For this review, take the finished solid that the model builds, in its own axes (mm). A direction names the side the tool comes from. Round coordinates to 2 decimals unless told otherwise and drop trailing zeros. Order: outer loops, then holes, each group sorted by start corner. A loop starts at its lowest first (then second) coordinate and runs counter-clockwise, first axis right, second up.
Autodesk Inventor part; units mm, degrees
ref_plane "Work Plane1" through (0, 98, 0) normal (0, -1, 0) x (1, 0, 0)
ref_plane "YZ Plane" through (0, 0, 0) normal (1, 0, 0) x (0, 1, 0)
ref_plane "XZ Plane" through (0, 0, 0) normal (0, 1, 0) x (-1, 0, 0)
sketch "Sketch1" plane through (0, 0, 0) normal (0, 1, 0) x (-1, 0, 0)
  line L0 (0, 0) -> (8, 0)
  line L1 (8, 0) -> (8, -120)
  line L2 (8, -120) -> (0, -120)
  line L3 (0, -120) -> (0, 0)
  line L4 (8, 0) -> (38, 0)
  line L5 (38, 0) -> (38, -120)
  line L6 (38, -120) -> (8, -120)
  line L7 (8, -120) -> (8, 0)
  circle A0 centre (20, -17) radius 2
  circle A1 centre (20, -30) radius 2
  circle A2 centre (20, -43) radius 2
  circle A3 centre (20, -77) radius 2
  circle A4 centre (20, -90) radius 2
  circle A5 centre (20, -103) radius 2
  circle A6 centre (30, -17) radius 2
  circle A7 centre (30, -30) radius 2
  circle A8 centre (30, -43) radius 2
  circle A9 centre (30, -77) radius 2
  circle A10 centre (30, -90) radius 2
  circle A11 centre (30, -103) radius 2
  dimension "d15" = 8
  dimension "d16" = 120
  dimension "d17" = 30
extrude "Extrusion3" add sketch "Sketch1" along normal blind 98 contours L0 L1 L2 L3
extrude "Extrusion4" add sketch "Sketch1" along normal blind 8 contours L4 L5 L6 L1
sketch "Sketch2" plane through (0, 0, 0) normal (1, 0, 0) x (0, 0, -1)
  line L0 (0, 0) -> (120, 0)
  line L1 (120, 0) -> (120, 98)
  line L2 (0, 0) -> (0, 35)
  line L3 (0, 8) -> (0, 98)
  circle A0 centre (25, 35) radius 2
  circle A1 centre (60, 35) radius 2
  dimension "d53" = 4
  dimension "d54" = 4
extrude "Extrusion5" cut sketch "Sketch2" against normal blind 10
ref_plane "Work Plane1" through (0, 98, 0) normal (0, -1, 0) x (1, 0, 0)
sketch "Sketch4" plane through (0, 98, 0) normal (0, -1, 0) x (1, 0, 0)
  line L0 (0, -120) -> (0, 0)
  line L1 (0, 0) -> (-8, 0)
  line L2 (-8, 0) -> (-8, -120)
  line L3 (-8, -120) -> (0, -120)
  line L4 (-8, 0) -> (-38, 0)
  line L5 (-38, 0) -> (-38, -120)
  line L6 (-38, -120) -> (-8, -120)
  line L7 (-8, -120) -> (-8, 0)
  circle A0 centre (-20, -17) radius 2
  circle A1 centre (-20, -30) radius 2
  circle A2 centre (-20, -43) radius 2
  circle A3 centre (-20, -77) radius 2
  circle A4 centre (-20, -90) radius 2
  circle A5 centre (-20, -103) radius 2
  circle A6 centre (-30, -77) radius 2
  circle A7 centre (-30, -90) radius 2
  circle A8 centre (-30, -103) radius 2
  circle A9 centre (-30, -43) radius 2
  circle A10 centre (-30, -30) radius 2
  circle A11 centre (-30, -17) radius 2
  point P0 (8, -120)
extrude "Extrusion6" add sketch "Sketch4" against normal blind 8
fillet "Fillet1" radius 4 6 edges at (-38, 102, 0) (-38, 102, -120) (-38, 4, -120) (-38, 4, 0) (-8, 98, -60) (-8, 8, -60)
properties part number "_3DPrint"
(1) Add section A-A on x = -14. Give the boundary of the cut face in (y, z), plus the area to 3 significant figures.
(2) Add section C-C on y = 35. Give the boundary of the cut face in (x, z).
(3) Add section B-B on z = -60. Give the boundary of the cut face in (x, y).
(4) Add section D-D on z = -30. Give the boundary of the cut face in (x, y).
(5) Draft analysis for pull direction X (two halves, no side actions). For faces 3 (the face through (-19, 106, -59)), 4 (the face through (-9.203, 96.859, -60.84)), 5 (the face through (-20, 102, -45)), state which applies: pulls with the +X half, pulls with the -X half, needs draft (parallel to the pull), parting line crosses it, or undercut.
(6) Tool access review of faces 1 (the face through (-30.923, 3.944, -28.226)), 2 (the face through (-8, 52, -59)): name each direction out of +Z, -Z, +X, -X, +Y, -Y from which nothing blocks a thin tool from reaching the whole face with its end or side.
(7) Wall thickness on L1, parallel to Y at x = -16, z = -77; L2, parallel to X at y = 78, z = -62.5; L3, parallel to X at y = 97.5, z = -73.5: over which ranges is each line inside the solid? List them lowest first.
Here are the results:
1. outline: (0, -120) - (8, -120) - (8, 0) - (0, 0) - close; (98, -120) - (106, -120) - (106, 0) - (98, 0) - close
1. area: 1,920 mm2
2. outline: (-8, -120) - (0, -120) - (0, -62) - (-8, -62) - close; (-8, -58) - (0, -58) - (0, -27) - (-8, -27) - close; (-8, -23) - (0, -23) - (0, 0) - (-8, 0) - close
3. outline: (-38, 0) - (0, 0) - (0, 33) - (-8, 33) - (-8, 12) arc R4 cw to (-12, 8) - (-38, 8) - close; (-38, 98) - (-12, 98) arc R4 cw to (-8, 94) - (-8, 37) - (0, 37) - (0, 106) - (-38, 106) - close
4. outline: (-38, 0) - (-32, 0) - (-32, 8) - (-38, 8) - close; (-38, 98) - (-32, 98) - (-32, 106) - (-38, 106) - close; (-28, 0) - (-22, 0) - (-22, 8) - (-28, 8) - close; (-28, 98) - (-22, 98) - (-22, 106) - (-28, 106) - close; (-18, 0) - (0, 0) - (0, 106) - (-18, 106) - (-18, 98) - (-12, 98) arc R4 cw to (-8, 94) - (-8, 12) arc R4 cw to (-12, 8) - (-18, 8) - close
5. face 3: needs draft
5. face 4: pulls with the -X half
5. face 5: undercut
6. face 1: +Y, -Y
6. face 2: +Z, -Z, -X
7. L1: y = 0 to 8, 98 to 106
7. L2: x = -8 to 0
7. L3: x = -10.06 to 0
